Geometry: see drawing. Coordinates: mm, zero at the bounding-box minimum. Give positions to 0.01 mm unless a question says otherwise; leave off trailing zeros. Loops run counter-clockwise (first coordinate to the right, second up) from the corner with the lowest first, then second, coordinate; pieces in that order, holes last. Notation, with made-up numbers: M -23,56 L 16,56 A17 cw 16,82 Z; hole C 80,2.25 d7. An arc over 180 degrees is marked long. Answer in a Markdown table with one row per item.
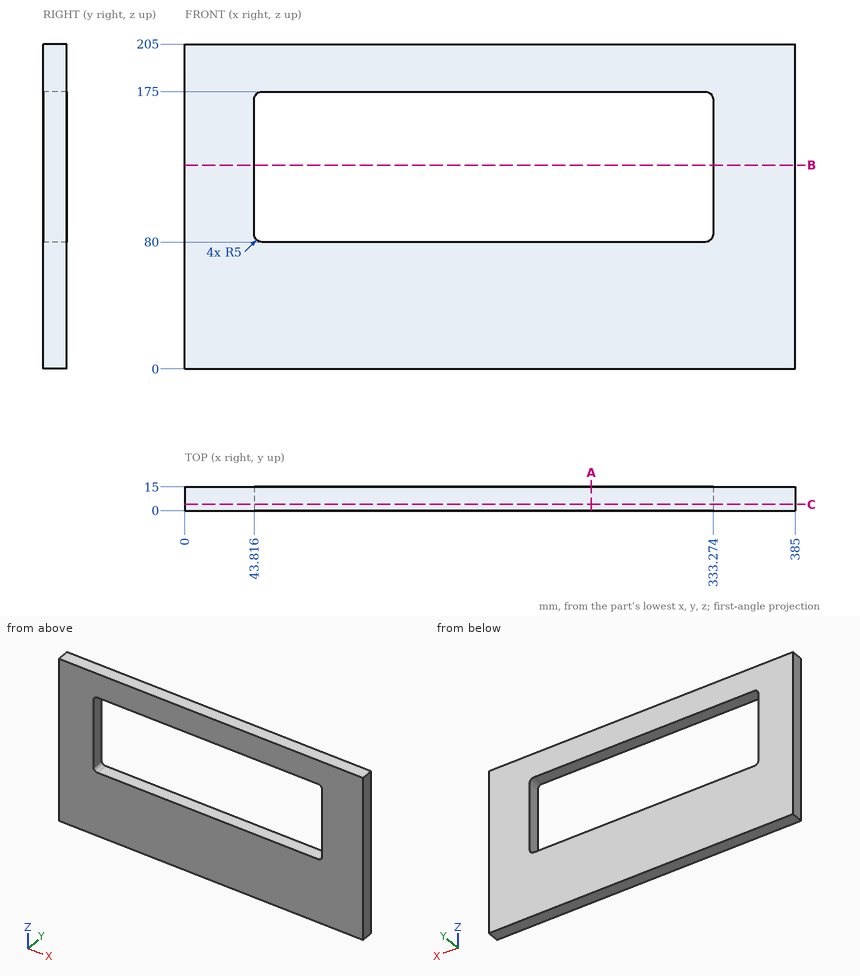
1) Section A-A, the plane x = 256.5. Return loops of the section in (y, z), then the cut area to 3 significant figures.
Reply:
| item | result |
|---|---|
| outline | M 0,0 L 15,0 L 15,80 L 0,80 Z; M 0,175 L 15,175 L 15,205 L 0,205 Z |
| area | 1,650 mm² |
2) Section C-C, the plane y = 4. Return loops of the section in (x, z).
Reply:
| item | result |
|---|---|
| outline | M 0,0 L 385,0 L 385,205 L 0,205 Z; hole M 43.82,85 A5 ccw 48.82,80 L 328.27,80 A5 ccw 333.27,85 L 333.27,170 A5 ccw 328.27,175 L 48.82,175 A5 ccw 43.82,170 Z |
3) Section B-B, the plane z = 128.5. Return loops of the section in (x, y).
Reply:
| item | result |
|---|---|
| outline | M 0,0 L 43.82,0 L 43.82,15 L 0,15 Z; M 333.27,0 L 385,0 L 385,15 L 333.27,15 Z |
4) Material intervals for L1, parallel to Z at x = 112, y = 9.25; L2, parallel to X at y = 1.5, z = 102; L3, parallel to Z at x = 48, y = 4, sorted ascending.
Reply:
| item | result |
|---|---|
| L1 | z = 0 to 80, 175 to 205 |
| L2 | x = 0 to 43.82, 333.27 to 385 |
| L3 | z = 0 to 80.07, 174.93 to 205 |
